```python
from build123d import *

# Parameters (mm, degrees)
SKETCH007_R    = 43
PAD002_DEPTH   = 7.75
SKETCH_R       = 5.5
HOLE001_DEPTH  = 15
HOLE001_TIPS_R = 5.5
SKETCH083_R    = 5.5
HOLE002_DEPTH  = 15
HOLE002_TIPS_R = 5.5


with BuildPart() as part:
    # Sketch007 → Pad002 (new body, symmetric)
    with BuildSketch(Plane.XY):
        with BuildLine():
            ThreePointArc((-15.28569, 49.702592), (-41.826163, 30.896149), (-52, 0))
            ThreePointArc((-52, 0), (-41.826156, -30.89613), (-15.285695, -49.702561))
            ThreePointArc((-11.831435, -53.613416), (-13.007952, -51.171659), (-15.285695, -49.702561))
            Line((-11.831435, -53.613416), (-10, -64))
            Line((-10, -64), (10, -64))
            Line((10, -64), (11.831435, -53.613416))
            ThreePointArc((15.285695, -49.702561), (13.007952, -51.171659), (11.831435, -53.613416))
            ThreePointArc((15.285695, -49.702561), (41.826156, -30.89613), (52, 0))
            ThreePointArc((52, 0), (41.826163, 30.896149), (15.28569, 49.702592))
            ThreePointArc((11.83143, 53.613447), (13.007947, 51.17169), (15.28569, 49.702592))
            Line((10, 64), (11.83143, 53.613447))
            Line((-10, 64), (10, 64))
            Line((-11.83143, 53.613447), (-10, 64))
            ThreePointArc((-15.28569, 49.702592), (-13.007947, 51.17169), (-11.83143, 53.613447))
        make_face()
        Circle(SKETCH007_R, mode=Mode.SUBTRACT)
    extrude(amount=PAD002_DEPTH, both=True)

    # Sketch (on Face6 of Pad002) → Hole001 (cut)
    with BuildSketch(Plane.XZ.offset(64)):
        Circle(SKETCH_R)
    extrude(amount=-HOLE001_DEPTH, mode=Mode.SUBTRACT)

    # Hole001 tips → Hole001 tip 1 section 0
    with BuildSketch(Plane.XZ.offset(49), mode=Mode.PRIVATE) as hole001_tip_1_s0:
        Circle(HOLE001_TIPS_R)
    loft([hole001_tip_1_s0.sketch, Vertex(0, -45.695267, 0)], mode=Mode.SUBTRACT)

    # Sketch083 (on Face7 of Hole001) → Hole002 (cut)
    with BuildSketch(Plane(origin=(0, 64, 0), x_dir=(-1, 0, 0), z_dir=(0, 1, 0))):
        Circle(SKETCH083_R)
    extrude(amount=-HOLE002_DEPTH, mode=Mode.SUBTRACT)

    # Hole002 tips → Hole002 tip 1 section 0
    with BuildSketch(Plane(origin=(0, 49, 0), x_dir=(-1, 0, 0), z_dir=(0, 1, 0)), mode=Mode.PRIVATE) as hole002_tip_1_s0:
        Circle(HOLE002_TIPS_R)
    loft([hole002_tip_1_s0.sketch, Vertex(0, 45.695267, 0)], mode=Mode.SUBTRACT)


solid = part.part
```
Design review of the part built by this model. Coordinates are the model's own, in mm. A direction names the side the tool comes from. Coordinates: 2 decimals unless noted, no trailing zeros. Loops run counter-clockwise (first coordinate to the right, second up) from the corner with the lowest first, then second, coordinate; pieces in that order, holes last. Notation, with made-up numbers: (-34.75, 54.25) -> (5.25, 54.25) arc R24 ccw to (5.25, 82.25) -> close; hole circle Ø6 at (37.5, -6.75). An arc over 180 degrees is marked (long way). Answer as a JSON object with one key per item and string values.
Q1. The part is to be moulded in two halves that separate along Z. For faces 1 (the flat face through (4, 43, -7.75)), 2 (the cylindrical face through (-12.983, -51.201, 0.109)), 3 (the cylindrical face through (-1.19, -56.6, -5.37)), say which applies: +Z half, -Z half, draft (parallel to the pull), parting line (faces both ways), or undercut.
Answer block:
{"face 1": "-Z half", "face 2": "draft", "face 3": "undercut"}
Q2. Clearance check with flat-ended pins moving along their axes: pin 1 Ø9 at (x, z) = (0, 0) entering from +Y; pin 2 Ø4 at (y, z) = (18.5, -1.5) entering from +X; pin 3 Ø2 at (y, z) = (11.5, -0.5) entering from +X. State where each tip first meets the part, or that it passes through.
Answer block:
{"pin 1": "stops at y = 48.4", "pin 2": "stops at x = 49.31", "pin 3": "stops at x = 50.93"}
Q3. Take a section at B-B on y = 18. Give the boundary of the cut face in (x, z).
Answer block:
{"outline": "(-48.79, -7.75) -> (-39.05, -7.75) -> (-39.05, 7.75) -> (-48.79, 7.75) -> close; (39.05, -7.75) -> (48.79, -7.75) -> (48.79, 7.75) -> (39.05, 7.75) -> close"}
Q4. To check wall thickness, follow L1, parallel to X at y = 0.5, z = 6.25; L2, parallel to Z at x = 0, y = 53; L3, parallel to Y at x = 25, z = -5.5. State the ranges of each line that lie inside material, in increasing order.
Answer block:
{"L1": "x = -52 to -43, 43 to 52", "L2": "z = -7.75 to -5.5, 5.5 to 7.75", "L3": "y = -45.6 to -34.99, 34.99 to 45.6"}
Q5. Take a section at A-A on x = 35.5. Give the boundary of the cut face in (y, z), plus the area to 3 significant figures.
Answer block:
{"outline": "(-38, -7.75) -> (-24.26, -7.75) -> (-24.26, 7.75) -> (-38, 7.75) -> close; (24.26, -7.75) -> (38, -7.75) -> (38, 7.75) -> (24.26, 7.75) -> close", "area": "426 mm^2"}
Q6. Tool access review of faces 4 (the flat face through (-10.93, -58.73, 0.11)), 5 (the cylindrical face through (1.19, 56.6, -5.37)): name each direction out of +Z, -Z, +X, -X, +Y, -Y from which nothing blocks a thin tool from reaching the whole face with its end or side.
Answer block:
{"face 4": "+Z, -Z, -X, -Y", "face 5": "+Y"}
